Verification items for this drawing (mm, ordinates from the low corner). A direction names the side the tool comes from. Round coordinates to 2 decimals unless told otherwise and drop trailing zeros. Write each loop counter-clockwise with the first axis right and the second up, starting at its lowest first coordinate (ties: lowest second). Pieces come first, ordered by that corner, then holes.
Item 1: Cross-section at D-D (z = 3.5). Enter the section's corners in (x, y), then the cut area to 3 significant figures.
Item 2: Cross-section at A-A (z = 16). Enter the section's corners in (x, y) (3 decimals), then the cut area to 3 significant figures.
Item 3: Cross-section at C-C (x = 28). Enter the section's corners in (y, z).
Item 4: Depth check by flat-ended pin: P1, Ø1.5, axis at x = 9, y = 3.5, coming from the -Z side; P2, Ø2.5, axis at y = 4, z = 2.5, coming from the -X side; P3, Ø2.5, axis at y = 1.5, z = 22.5, coming from the -X side. Enter the tip coordinate at first touch or a pass-through.
Item 5: Access from +Z, -Z, +X, -X, +Y, -Y to the whole of each face (thin tool, end or side, straight path). Record for the marked faces 1, 2 and 3.
Item 6: Draft check along Z on the marked faces 4, 5, 6 and 7. Enter one of: pulls with the +Z half, pulls with the -Z half, needs draft (parallel to the pull), parting line crosses it, or undercut.
Item 7: Cross-section at B-B (y = 3.65). Enter the section's corners in (x, z) (3 decimals), then the cut area to 3 significant figures.
Item 8: Scan lines: probe 1 along X at (y, z) = (4.4, 16) (3 decimals); probe 2 along Z at (x, y) = (27, 1.5); probe 3 along X at (y, z) = (4.95, 2). Record each from-to range of solid material in increasing order.
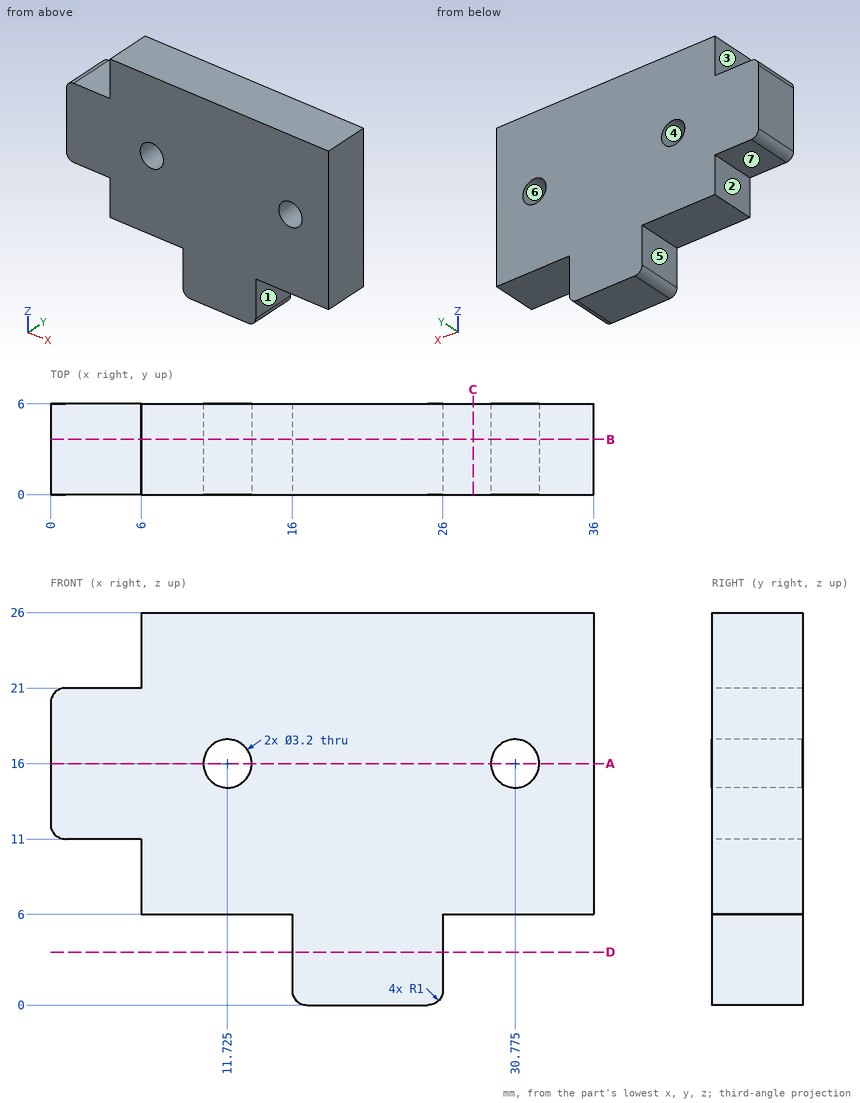
Resolved:
1. outline: (16, 0) - (26, 0) - (26, 6) - (16, 6) - close
1. area: 60.0 mm2
2. outline: (0, 0) - (10.125, 0) - (10.125, 6) - (0, 6) - close; (13.325, 0) - (29.175, 0) - (29.175, 6) - (13.325, 6) - close; (32.375, 0) - (36, 0) - (36, 6) - (32.375, 6) - close
2. area: 178 mm2
3. outline: (0, 6) - (6, 6) - (6, 26) - (0, 26) - close
4. P1: stops at z = 6
4. P2: stops at x = 16
4. P3: stops at x = 6
5. face 1: -Z, +X, +Y, -Y
5. face 2: -Z, -X, +Y, -Y
5. face 3: +Z, -X, +Y, -Y
6. face 4: undercut
6. face 5: needs draft
6. face 6: undercut
6. face 7: pulls with the -Z half
7. outline: (0, 12) arc R1 ccw to (1, 11) - (6, 11) - (6, 6) - (16, 6) - (16, 1) arc R1 ccw to (17, 0) - (25, 0) arc R1 ccw to (26, 1) - (26, 6) - (36, 6) - (36, 26) - (6, 26) - (6, 21) - (1, 21) arc R1 ccw to (0, 20) - close; hole circle Ø3.2 at (11.725, 16); hole circle Ø3.2 at (30.775, 16)
7. area: 703 mm2
8. probe 1: x = 0 to 10.125, 13.325 to 29.175, 32.375 to 36
8. probe 2: z = 6 to 26
8. probe 3: x = 16 to 26
